```python
from build123d import *

# Parameters (mm, degrees)
F1_DEPTH = 1955.8
F2_SIZE2 = 32.5105174577
F2_SIZE  = 25.4
F4_DEPTH = 76.201


# Not quite as in the source:
# - a feature names something its author has since deleted; it is built from what else it names


with BuildPart() as f1:
    # F0 (on Right) → F1 (new body)
    with BuildSketch(Plane.YZ):
        with BuildLine():
            Line((0, 0), (0, -25.4))
            Line((0, -25.4), (25.4, -25.4))
            Line((25.4, -25.4), (25.4, -19.05))
            Line((25.4, -19.05), (50.8, -19.05))
            Line((50.8, -19.05), (50.8, -25.4))
            Line((50.8, -25.4), (76.2, -25.4))
            Line((76.2, -25.4), (76.2, 0))
            ThreePointArc((76.2, 0), (38.1, 38.1), (0, 0))
        make_face()
    extrude(amount=F1_DEPTH)

    # F2
    f2_edges = [f1.edges().sort_by_distance(p)[0] for p in [
        (0, 12.7, -25.4),
    ]]
    f2_side = f1.faces().sort_by_distance((977.9, 12.7, -25.4))[0]
    chamfer(f2_edges, length=F2_SIZE, length2=F2_SIZE2, reference=f2_side)

    # F3 (on Front) → F4 (cut, through all)
    with BuildSketch(Plane.XZ):
        Polygon((44.9116937816, 39.251241833), (17.98238638, 50.449128889), (0, 45.5416738987), (0, 7.1105174577), align=None)
    extrude(amount=-F4_DEPTH, mode=Mode.SUBTRACT)


solid = f1.part
```
Here's how the part is built. I have some questions about the finished solid (model axes, mm). Round coordinates to 2 decimals unless told otherwise and drop trailing zeros. Order: outer loops, then holes, each group sorted by start corner. A loop starts at its lowest first (then second) coordinate and runs counter-clockwise, first axis right, second up. Notation, with made-up numbers: (-38.5, -13) -> (-21.5, -13) arc R12 ccw to (-21.5, 6) -> close; hole circle Ø3 at (37, 85). An arc over 180 degrees is marked (long way). Use a Markdown table: item, result. Add a question column.
(1) Suppose I cut it at B-B, the plane y = 38.1. Please give me the cut outline in (x, z), and give its area (3 significant figures).
(2) Suppose I cut it at A-A, the plane x = 1266.5. Please give me the cut outline in (y, z), and give its area (3 significant figures).
(3) For pin 1 Ø7.5 at (x, y) = (1391.5, 33) entering from -Z; pin 2 Ø6 at (x, y) = (1469.5, 12) entering from +Z; pin 3 Ø1.5 at (x, y) = (714.5, 21) entering from +Z, each with a flat end and sliding along its axis, tell me the tip position at first contact or that it passes through.
(4) I need wall thicknesses on line 1 along Z through (x, y) = (523, 33.5); line 2 along Z through (x, y) = (1320, 6); line 3 along Y through (x, z) = (1477, 7). Which ranges of each line are inside material? Lowest first, please.
Verdict:
| question | item | result |
|---|---|---|
| 1 | outline | (0, 7.11) -> (20.44, -19.05) -> (1955.8, -19.05) -> (1955.8, 38.1) -> (43.3, 38.1) -> close |
| 1 | area | 111,000 mm2 |
| 2 | outline | (0, -25.4) -> (25.4, -25.4) -> (25.4, -19.05) -> (50.8, -19.05) -> (50.8, -25.4) -> (76.2, -25.4) -> (76.2, 0) arc R38.1 ccw to (0, 0) -> close |
| 2 | area | 4,050 mm2 |
| 3 | pin 1 | z = -19.05 |
| 3 | pin 2 | z = 30.3 |
| 3 | pin 3 | z = 34.41 |
| 4 | line 1 | -19.05 to 37.82 |
| 4 | line 2 | -25.4 to 20.52 |
| 4 | line 3 | 0.65 to 75.55 |
